Check sheet for the modelled part. Datum: model origin and axes. Units: mm. Coordinates: 2 decimals unless noted, no trailing zeros. Write each loop counter-clockwise with the first axis right and the second up, starting at its lowest first coordinate (ties: lowest second). Pieces come first, ordered by that corner, then holes. Notation, with made-up numbers: M 13.25,62 L 51.25,62 A7 ccw 51.25,69 Z; hole C 76.5,72.5 d11. An arc over 180 degrees is marked long. Answer as CSV lines item,"result". Start each with the question number.
1) Material ranges on L1, parallel to Z at x = 0.5, y = -16.5; L2, parallel to Z at x = -5.5, y = -14.25; L3, parallel to X at y = -13, z = -1.5, recorded low to high. Write a range as [from, to].
2) Section check C-C (y = -12.75). Record the cut outline in (x, z), and give its area (3 significant figures).
3) Draft check along X on faces 1 (the cylindrical face through (12.115, -9.392, 3.813)), 2 (the cylindrical face through (-55.837, -9.392, -3.866)), 3 (the cylindrical face through (24.7, -9.39, -25.27)), 4 (the cylindrical face through (-25.27, -9.392, -24.696)). Enter one of: +X half, -X half, draft (parallel to the pull), parting line (faces both ways), or undercut.
4) Section check B-B (z = 11). Record the cut outline in (x, y), and give its area (3 significant figures).
5) Go/stop test with flat-tipped pins: pin 1 Ø3 at (y, z) = (-8.5, -27.5) entering from +X; pin 2 Ø1.5 at (x, z) = (-16.5, -40) entering from +Y; pin 3 Ø4 at (y, z) = (-12.5, -7) entering from +X; pin 4 Ø6 at (y, z) = (-13.5, 21.5) entering from +X. Record where each tip stops, or that it passes through.
6) Section check A-A (x = 49). Record the cut outline in (y, z).
7) Section check D-D (z = -2). Record the cut outline in (x, y), and give its area (3 significant figures).
from build123d import *

# Parameters (mm, degrees)
F0_R     = 6.35
F0_R_2   = 12.7
F1_DEPTH = 19.05


with BuildPart() as f1:
    # F0 (on Front) → F1 (new body)
    with BuildSketch(Plane.XZ):
        with BuildLine():
            ThreePointArc((-12.69828, 50.798278), (-25.024948, 25.024947), (-50.79828, 12.698278))
            ThreePointArc((-50.79828, 12.698278), (-63.49828, -0.001722), (-50.79828, -12.701722))
            ThreePointArc((-50.79828, -12.701722), (-24.980044, -24.983485), (-12.69828, -50.801722))
            ThreePointArc((-12.69828, -50.801722), (0.00172, -63.501722), (12.70172, -50.801722))
            ThreePointArc((12.70172, -50.801722), (24.983496, -24.983498), (50.80172, -12.701722))
            ThreePointArc((50.80172, -12.701722), (63.50172, -0.001722), (50.80172, 12.698278))
            ThreePointArc((50.80172, 12.698278), (24.983506, 24.980065), (12.70172, 50.798278))
            ThreePointArc((12.70172, 50.798278), (0.00172, 63.498278), (-12.69828, 50.798278))
        make_face()
        with Locations((0.00172, -50.801722)):
            Circle(F0_R, mode=Mode.SUBTRACT)
        with Locations((-50.79828, -0.001722)):
            Circle(F0_R, mode=Mode.SUBTRACT)
        with Locations((0.00172, -0.001722)):
            Circle(F0_R_2, mode=Mode.SUBTRACT)
        with Locations((0.00172, 50.798278)):
            Circle(F0_R, mode=Mode.SUBTRACT)
        with Locations((50.80172, -0.001722)):
            Circle(F0_R, mode=Mode.SUBTRACT)
    extrude(amount=F1_DEPTH)


solid = f1.part
Results found:
1,L1,"z = [-63.49, -57.13], [-44.47, -12.69], [12.69, 44.47], [57.13, 63.49]"
1,L2,"z = [-62.25, -53.97], [-47.63, -11.45], [11.44, 47.63], [53.97, 62.24]"
1,L3,"x = [-63.41, -56.97], [-44.63, -12.61], [12.61, 44.63], [56.97, 63.41]"
2,outline,"M -50.8,-12.7 A42.7 cw -12.7,-50.8 A12.7 ccw 12.7,-50.8 A42.7 cw 50.8,-12.7 A12.7 ccw 50.8,12.7 A42.7 cw 12.7,50.8 A12.7 ccw -12.7,50.8 A42.92 cw -50.8,12.7 A12.7 ccw Z; hole C -50.8,0 d12.7; hole C 0,0 d25.4; hole C 0,-50.8 d12.7; hole C 0,50.8 d12.7; hole C 50.8,0 d12.7"
2,area,"6,010 mm2"
3,face 1,"undercut"
3,face 2,"undercut"
3,face 3,"+X half"
3,face 4,"-X half"
4,outline,"M -57.14,-19.05 L -6.34,-19.05 L -6.34,0 L -57.14,0 Z; M 6.35,-19.05 L 57.15,-19.05 L 57.15,0 L 6.35,0 Z"
4,area,"1,940 mm2"
5,pin 1,"stops at x = 24"
5,pin 2,"passes through"
5,pin 3,"stops at x = 62.48"
5,pin 4,"stops at x = 33.31"
6,outline,"M -19.05,-12.93 L 0,-12.93 L 0,-6.09 L -19.05,-6.09 Z; M -19.05,6.09 L 0,6.09 L 0,12.92 L -19.05,12.92 Z"
7,outline,"M -63.34,-19.05 L -56.83,-19.05 L -56.83,0 L -63.34,0 Z; M -44.77,-19.05 L -12.54,-19.05 L -12.54,0 L -44.77,0 Z; M 12.54,-19.05 L 44.77,-19.05 L 44.77,0 L 12.54,0 Z; M 56.83,-19.05 L 63.34,-19.05 L 63.34,0 L 56.83,0 Z"
7,area,"1,480 mm2"
